Answer from the drawing. Dimensions are ordinates in mm from the lowest x, y and z of the part. A direction names the side the tool comes from. Round coordinates to 2 decimals unless told otherwise and drop trailing zeros. Write each loop counter-clockwise with the first axis right and the second up, starting at its lowest first coordinate (ties: lowest second). Pieces come first, ordered by that corner, then holes. Notation, with made-up numbers: (78.5, -19) - (101.5, -19) arc R10 ccw to (101.5, -14) - close; hole circle Ø10 at (70, 12). An arc over 180 degrees is marked (long way). Answer as a JSON object with one key per item and string values.
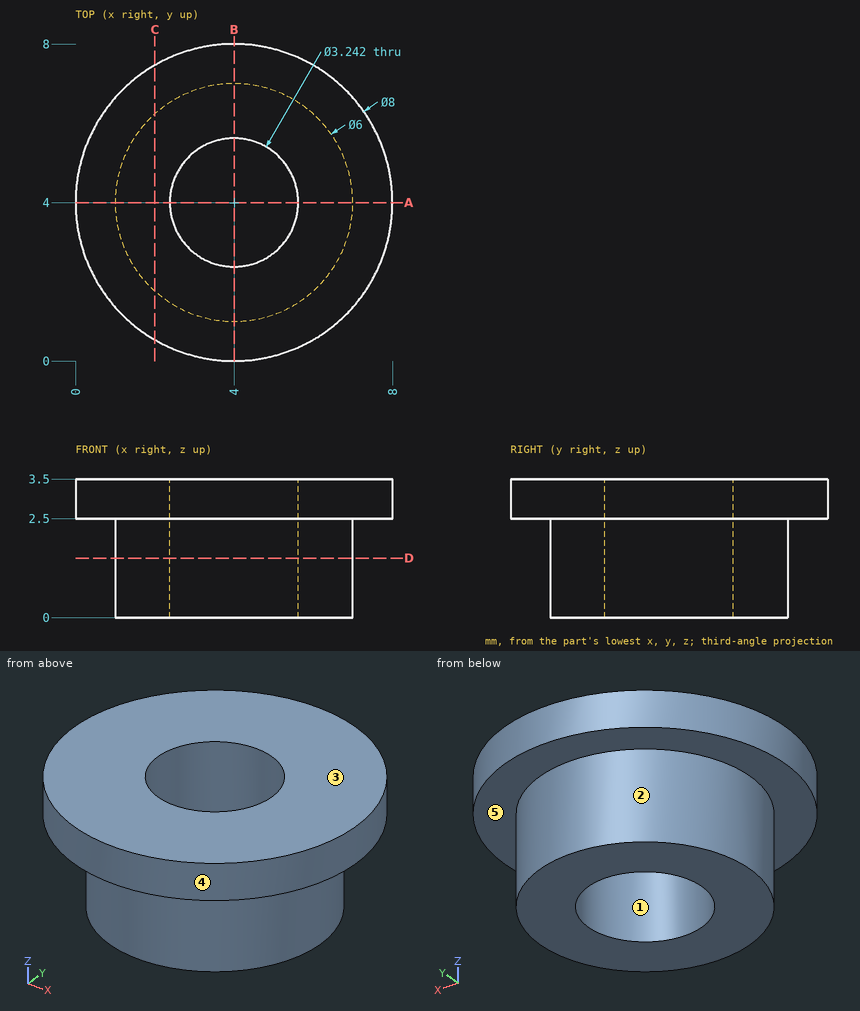
Item 1: A cutting plane is placed at D-D (z = 1.5). Write down the section's boundary in (x, y).
Results found:
{"outline": "circle Ø6 at (4, 4); hole circle Ø3.24 at (4, 4)"}
Item 2: A cutting plane is placed at A-A (y = 4). Write down the section's boundary in (x, z), and give its area (3 significant figures).
Results found:
{"outline": "(0, 2.5) - (1, 2.5) - (1, 0) - (2.38, 0) - (2.38, 3.5) - (0, 3.5) - close; (5.62, 0) - (7, 0) - (7, 2.5) - (8, 2.5) - (8, 3.5) - (5.62, 3.5) - close", "area": "11.7 mm²"}
Item 3: For the marked faces 4 and 5, determine the directions among +Z, -Z, +X, -X, +Y, -Y from which every point of the face is accessible in a straight line to the end or side of a thin tool.
Results found:
{"face 4": "+Z, -Z", "face 5": "-Z"}
Item 4: A cutting plane is placed at C-C (x = 2). Write down the section's boundary in (y, z).
Results found:
{"outline": "(0.54, 2.5) - (1.76, 2.5) - (1.76, 0) - (6.24, 0) - (6.24, 2.5) - (7.46, 2.5) - (7.46, 3.5) - (0.54, 3.5) - close"}
Item 5: Consider line 1 along Y through (x, z) = (4, 1.85); line 2 along Z through (x, y) = (1.75, 6.5); line 3 along X through (y, z) = (4.5, 2.3). Determine where each line is inside the solid, lowest interval first.
Results found:
{"line 1": "1 to 2.38, 5.62 to 7", "line 2": "2.5 to 3.5", "line 3": "1.04 to 2.46, 5.54 to 6.96"}
Item 6: Determine the mould class of the marked faces 1, 2 and 3 for opening direction X: pulls with the +X half, pulls with the -X half, needs draft (parallel to the pull), parting line crosses it, or undercut.
Results found:
{"face 1": "undercut", "face 2": "parting line crosses it", "face 3": "needs draft"}
Item 7: Each of these flat-tipped pins is pushed along its axis until it touches: P1, Ø2, axis at x = 5.5, z = 3, coming from the +Y side; P2, Ø2, axis at y = 2, z = 2, coming from the +X side. Where does it stop, or does it pass through?
Results found:
{"P1": "y = 7.97", "P2": "x = 7.84"}
